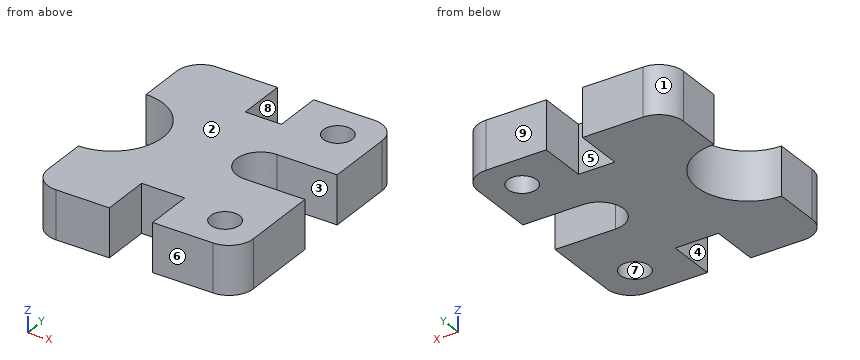
from build123d import *

# Parameters (mm, degrees)
SKETCH1_R           = 6
BOSS_EXTRUDE1_DEPTH = 20


with BuildPart() as part:
    # Sketch1 → Boss-Extrude1 (new body)
    with BuildSketch(Plane.XY):
        with BuildLine():
            Line((-7.5, 50), (-7.5, 30))
            Line((-7.5, 30), (7.5, 30))
            Line((7.5, 30), (7.5, 50))
            Line((7.5, 50), (32.5, 50))
            ThreePointArc((32.5, 50), (39.571067812, 47.071067812), (42.5, 40))
            Line((42.5, 40), (42.5, 12.097843739))
            Line((42.5, 12.097843739), (17.5, 12.097843739))
            ThreePointArc((17.5, 12.097843739), (7.5, 2.097843739), (17.5, -7.902156261))
            Line((17.5, -7.902156261), (42.5, -7.902156261))
            Line((42.5, -7.902156261), (42.5, -40))
            ThreePointArc((42.5, -40), (39.571067812, -47.071067812), (32.5, -50))
            Line((32.5, -50), (7.5, -50))
            Line((7.5, -50), (7.5, -30))
            Line((7.5, -30), (-10.372609166, -30))
            Line((-10.372609166, -30), (-10.372609166, -50))
            Line((-10.372609166, -50), (-32.5, -50))
            ThreePointArc((-32.5, -50), (-39.571067812, -47.071067812), (-42.5, -40))
            Line((-42.5, -40), (-42.5, -21))
            ThreePointArc((-42.5, -21), (-21.5, 0), (-42.5, 21))
            Line((-42.5, 21), (-42.5, 40))
            ThreePointArc((-42.5, 40), (-39.571067812, 47.071067812), (-32.5, 50))
            Line((-32.5, 50), (-7.5, 50))
        make_face()
        with Locations((27.5, 35)):
            Circle(SKETCH1_R, mode=Mode.SUBTRACT)
        with Locations((27.5, -35)):
            Circle(SKETCH1_R, mode=Mode.SUBTRACT)
    extrude(amount=BOSS_EXTRUDE1_DEPTH)


solid = part.part
The model under review builds one solid part; all positions refer to its coordinate system, in mm. Face numbers are marked on the shaded views. A direction names the side the tool comes from. Coordinates: 2 decimals unless noted, no trailing zeros. Write each loop counter-clockwise with the first axis right and the second up, starting at its lowest first coordinate (ties: lowest second). Pieces come first, ordered by that corner, then holes. Notation, with made-up numbers: (19, 56) - (37, 56) arc R30 ccw to (37, 79) - close; hole circle Ø6 at (-39, 19). An arc over 180 degrees is marked (long way). Answer as a JSON object with one key per item and string values. Group by question number.
1. Add section A-A (y = -35). Give the boundary of the cut face in (x, z).
2. Mouldability with a two-part tool opening along Y and no side actions: class the marked faces 6, 7, 8 and 9 as pulls with the +Y half, pulls with the -Y half, needs draft (parallel to the pull), parting line crosses it, or undercut.
3. Clearance check with a flat-ended pin moving along its axis: pin 1 Ø2 at (y, z) = (5.5, 14.5) entering from -X. State where the tip first meets the part, or that it passes through.
4. To check wall thickness, follow probe 1 along Y at (x, z) = (27.5, 4.75); probe 2 along Y at (x, z) = (22, 15.5); probe 3 along Y at (x, z) = (17.5, 1.75). State the ranges of each line that lie inside material, in increasing order.
5. Add section C-C (x = -34). Give the boundary of the cut face in (y, z), plus the area to 3 significant figures.
6. Add section B-B (z = 10.75). Give the boundary of the cut face in (x, y).
7. Add section D-D (x = 27.5). Give the boundary of the cut face in (y, z), plus the area to 3 significant figures.
8. Machinability: for the marked faces 1, 2, 3, 4 and 5, which of the approach directions +Z, -Z, +X, -X, +Y, -Y give a long, thin tool a straight path to every point of the face, cutting with its end or side? Answer none if there is none.
Findings:
{
 "1": {"outline": "(-42.5, 0) - (-10.37, 0) - (-10.37, 20) - (-42.5, 20) - close; (7.5, 0) - (21.5, 0) - (21.5, 20) - (7.5, 20) - close; (33.5, 0) - (42.5, 0) - (42.5, 20) - (33.5, 20) - close"},
 "2": {"face 6": "pulls with the -Y half", "face 7": "undercut", "face 8": "needs draft", "face 9": "pulls with the +Y half"},
 "3": {"pin 1": "x = -22.53"},
 "4": {"probe 1": "-50 to -41, -29 to -7.9, 12.1 to 29, 41 to 50", "probe 2": "-50 to -37.4, -32.6 to -7.9, 12.1 to 32.6, 37.4 to 50", "probe 3": "-50 to -7.9, 12.1 to 50"},
 "5": {"outline": "(-49.89, 0) - (-19.2, 0) - (-19.2, 20) - (-49.89, 20) - close; (19.2, 0) - (49.89, 0) - (49.89, 20) - (19.2, 20) - close", "area": "1,230 mm²"},
 "6": {"outline": "(-42.5, -40) arc R10 ccw to (-32.5, -50) - (-10.37, -50) - (-10.37, -30) - (7.5, -30) - (7.5, -50) - (32.5, -50) arc R10 ccw to (42.5, -40) - (42.5, -7.9) - (17.5, -7.9) arc R10 cw to (17.5, 12.1) - (42.5, 12.1) - (42.5, 40) arc R10 ccw to (32.5, 50) - (7.5, 50) - (7.5, 30) - (-7.5, 30) - (-7.5, 50) - (-32.5, 50) arc R10 ccw to (-42.5, 40) - (-42.5, 21) arc R21 cw to (-42.5, -21) - close; hole circle Ø12 at (27.5, -35); hole circle Ø12 at (27.5, 35)"},
 "7": {"outline": "(-50, 0) - (-41, 0) - (-41, 20) - (-50, 20) - close; (-29, 0) - (-7.9, 0) - (-7.9, 20) - (-29, 20) - close; (12.1, 0) - (29, 0) - (29, 20) - (12.1, 20) - close; (41, 0) - (50, 0) - (50, 20) - (41, 20) - close", "area": "1,120 mm²"},
 "8": {"face 1": "+Z, -Z, -X, +Y", "face 2": "+Z, +X, -X, +Y, -Y", "face 3": "+Z, -Z, +X", "face 4": "+Z, -Z, -Y", "face 5": "+Z, -Z, +Y"}
}
